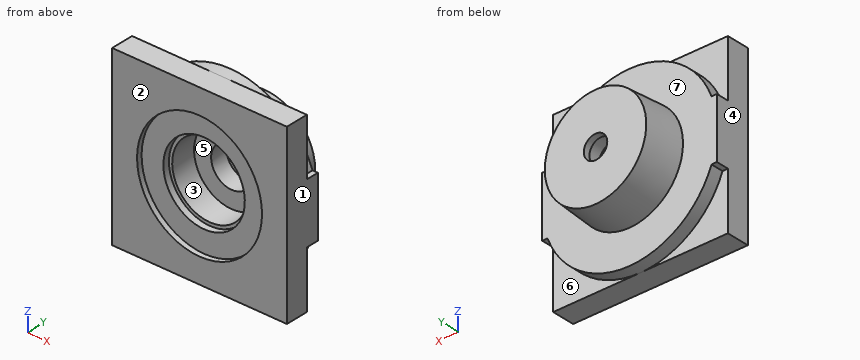
```python
from build123d import *

# Parameters (mm, degrees)
SKETCH1_W               = 7.01
SKETCH1_H               = 7.01
BOSS_EXTRUDE1_DEPTH     = 0.92
SKETCH2_R               = 3.505
BOSS_EXTRUDE2_DEPTH     = 0.83
SKETCH3_R               = 2.135
BOSS_EXTRUDE3_DEPTH     = 1.752116255
SKETCH4_R               = 2.085
CUT_EXTRUDE1_DEPTH      = 1
CUT_EXTRUDE2_DEPTH      = 7.069173606
CUT_EXTRUDE2_DEPTH_BACK = 7.069173606
SKETCH5_W               = 2.65
SKETCH5_H               = 2.65
SKETCH6_W               = 8.843273239
SKETCH6_H               = 10.721573241
SKETCH6_W_2             = 7.01
SKETCH6_H_2             = 7.01
SKETCH6_W_3             = 6
SKETCH6_H_3             = 6
CUT_EXTRUDE3_DEPTH      = 10
SKETCH7_W               = 8.855260717
SKETCH7_H               = 9.729262333
SKETCH7_R               = 3
CUT_EXTRUDE4_DEPTH      = 0.83
SKETCH8_W               = 2.771053774
SKETCH8_H               = 2.773686404
BOSS_EXTRUDE4_DEPTH     = 2.502116255
SKETCH9_R               = 0.554
CUT_EXTRUDE5_DEPTH      = 0.3
SKETCH10_R              = 0.47
CUT_EXTRUDE6_DEPTH      = 100
SKETCH11_R              = 1.501
CUT_EXTRUDE7_DEPTH      = 0.48
SKETCH12_R              = 0.817
CUT_EXTRUDE8_DEPTH      = 0.7
SKETCH14_R              = 0.582
CUT_EXTRUDE9_DEPTH      = 0.56
BOSS_EXTRUDE5_START     = 0.05
SKETCH15_R              = 0.554
SKETCH15_R_2            = 0.47
BOSS_EXTRUDE5_DEPTH     = 0.05
BOSS_EXTRUDE6_START     = 0.79
SKETCH16_R              = 2.085
SKETCH16_R_2            = 1.63
BOSS_EXTRUDE6_DEPTH     = 0.79
BOSS_EXTRUDE7_START     = 0.53
SKETCH17_R              = 1.63
SKETCH17_R_2            = 1.501
BOSS_EXTRUDE7_DEPTH     = 0.53
SKETCH18_R              = 2.572537364
SKETCH18_R_2            = 1.5
CUT_EXTRUDE10_DEPTH     = 1.752116255
BOSS_EXTRUDE8_START     = 0.21
SKETCH19_R              = 2.085
SKETCH19_R_2            = 1.705
BOSS_EXTRUDE8_DEPTH     = 0.21
SKETCH20_W              = 6.707027697
SKETCH20_H              = 11.442069063
SKETCH20_R              = 1.8
CUT_EXTRUDE11_DEPTH     = 0.83
SKETCH21_W              = 6.520255289
SKETCH21_H              = 15.458610975
SKETCH21_W_2            = 3.8
SKETCH21_H_2            = 3.8
CUT_EXTRUDE12_DEPTH     = 10
SKETCH23_W              = 6.99
SKETCH23_H              = 6.99
SKETCH23_W_2            = 3.502421246
SKETCH23_H_2            = 3.548313749
BOSS_EXTRUDE9_DEPTH     = 0.92
SKETCH24_W              = 6.057488838
SKETCH24_H              = 5.341048382
CUT_EXTRUDE14_DEPTH     = 0.13
SKETCH25_R              = 3.495
SKETCH25_R_2            = 1.679124266
BOSS_EXTRUDE10_DEPTH    = 0.83
SKETCH26_W              = 0.8
SKETCH26_H              = 2.36
BOSS_EXTRUDE11_DEPTH    = 0.83
SKETCH27_W              = 0.802423375
SKETCH27_H              = 2.36
BOSS_EXTRUDE12_DEPTH    = 0.83
SKETCH28_R              = 2.14
SKETCH28_R_2            = 1.325961915
BOSS_EXTRUDE13_DEPTH    = 1.622116255
SKETCH29_R              = 2.5
CUT_EXTRUDE15_DEPTH     = 0.21
SKETCH30_W              = 0.025
SKETCH30_H              = 0.83
BOSS_EXTRUDE14_DEPTH    = 0.4
SKETCH31_W              = 0.025
SKETCH31_H              = 0.83
BOSS_EXTRUDE15_DEPTH    = 0.4
SKETCH32_R              = 5.119404283
SKETCH32_R_2            = 2.14
CUT_EXTRUDE16_DEPTH     = 0.32
SKETCH33_W              = 6.584709795
SKETCH33_H              = 4.796866642
CUT_EXTRUDE17_DEPTH     = 0.37
SKETCH35_W              = 5.183427323
SKETCH35_H              = 5.029681598
SKETCH35_R              = 2.14
CUT_EXTRUDE18_DEPTH     = 1.572116
CUT_EXTRUDE18_DRAFT     = -4


with BuildPart() as part:
    # Sketch1 → Boss-Extrude1 (new body)
    with BuildSketch(Plane(origin=(0, 0, 0), x_dir=(1, 0, 0), z_dir=(0, 1, 0))):
        Rectangle(SKETCH1_W, SKETCH1_H)
    extrude(amount=BOSS_EXTRUDE1_DEPTH)

    # Sketch2 → Boss-Extrude2 (add)
    with BuildSketch(Plane(origin=(0, 0.92, 0), x_dir=(1, 0, 0), z_dir=(0, 1, 0))):
        with Locations(Location((0, 0, 0), (0, 0, 270))):
            Circle(SKETCH2_R)
    extrude(amount=BOSS_EXTRUDE2_DEPTH)

    # Sketch3 → Boss-Extrude3 (add)
    with BuildSketch(Plane(origin=(0, 1.75, 0), x_dir=(1, 0, 0), z_dir=(0, 1, 0))):
        with Locations(Location((0, 0, 0), (0, 0, 270))):
            Circle(SKETCH3_R)
    extrude(amount=BOSS_EXTRUDE3_DEPTH)

    # Sketch4 → Cut-Extrude1 (cut)
    with BuildSketch(Plane.XZ):
        with Locations(Location((0, 0, 0), (0, 0, 270))):
            Circle(SKETCH4_R)
    extrude(amount=-CUT_EXTRUDE1_DEPTH, mode=Mode.SUBTRACT)

    # Sketch5 → Cut-Extrude2 (cut, two sides: drawn at the far end of the back side and taken through both)
    with BuildSketch(Plane(origin=(0, 3.502116255, 0), x_dir=(1, 0, 0), z_dir=(0, 1, 0)).offset(-CUT_EXTRUDE2_DEPTH_BACK)):
        Rectangle(SKETCH5_W, SKETCH5_H)
    extrude(amount=CUT_EXTRUDE2_DEPTH + CUT_EXTRUDE2_DEPTH_BACK, mode=Mode.SUBTRACT)

    # Sketch6 → Cut-Extrude3 (cut)
    # profile 1 of 2: a face of its own
    with BuildSketch(Plane.XZ):
        with Locations((-0.050657098, -0.002715124)):
            Rectangle(SKETCH6_W, SKETCH6_H)
        Rectangle(SKETCH6_W_2, SKETCH6_H_2, mode=Mode.SUBTRACT)
    # profile 2 of 2: a face of its own
    with BuildSketch(Plane.XZ):
        Rectangle(SKETCH6_W_2, SKETCH6_H_2)
        Rectangle(SKETCH6_W_3, SKETCH6_H_3, mode=Mode.SUBTRACT)
    extrude(amount=-CUT_EXTRUDE3_DEPTH, mode=Mode.SUBTRACT)

    # Sketch7 → Cut-Extrude4 (cut)
    with BuildSketch(Plane(origin=(0, 1.75, 0), x_dir=(1, 0, 0), z_dir=(0, 1, 0))):
        with Locations((-0.111516438, -0.542198567)):
            Rectangle(SKETCH7_W, SKETCH7_H)
        with Locations(Location((0, 0, 0), (0, 0, 270))):
            Circle(SKETCH7_R, mode=Mode.SUBTRACT)
    extrude(amount=-CUT_EXTRUDE4_DEPTH, mode=Mode.SUBTRACT)

    # Sketch8 → Boss-Extrude4 (add)
    with BuildSketch(Plane.XZ.offset(-1)):
        with Locations((0.002668444, 0.023551669)):
            Rectangle(SKETCH8_W, SKETCH8_H)
    extrude(amount=-BOSS_EXTRUDE4_DEPTH)

    # Sketch9 → Cut-Extrude5 (cut)
    with BuildSketch(Plane(origin=(0, 3.502116255, 0), x_dir=(1, 0, 0), z_dir=(0, 1, 0))):
        with Locations(Location((0, 0, 0), (0, 0, 270))):
            Circle(SKETCH9_R)
    extrude(amount=-CUT_EXTRUDE5_DEPTH, mode=Mode.SUBTRACT)

    # Sketch10 → Cut-Extrude6 (cut)
    with BuildSketch(Plane(origin=(0, 3.202116255, 0), x_dir=(1, 0, 0), z_dir=(0, 1, 0))):
        with Locations(Location((0, 0, 0), (0, 0, 270))):
            Circle(SKETCH10_R)
    extrude(amount=-CUT_EXTRUDE6_DEPTH, mode=Mode.SUBTRACT)

    # Sketch11 → Cut-Extrude7 (cut)
    with BuildSketch(Plane.XZ.offset(-1)):
        with Locations(Location((0, 0, 0), (0, 0, 270))):
            Circle(SKETCH11_R)
    extrude(amount=-CUT_EXTRUDE7_DEPTH, mode=Mode.SUBTRACT)

    # Sketch12 → Cut-Extrude8 (cut)
    with BuildSketch(Plane.XZ.offset(-1.48)):
        with Locations(Location((0, 0, 0), (0, 0, 270))):
            Circle(SKETCH12_R)
    extrude(amount=-CUT_EXTRUDE8_DEPTH, mode=Mode.SUBTRACT)

    # Sketch14 → Cut-Extrude9 (cut)
    with BuildSketch(Plane.XZ.offset(-2.18)):
        with Locations(Location((0, 0, 0), (0, 0, 270))):
            Circle(SKETCH14_R)
    extrude(amount=-CUT_EXTRUDE9_DEPTH, mode=Mode.SUBTRACT)

    # Sketch15 → Boss-Extrude5 (add)
    with BuildSketch(Plane(origin=(0, 3.202116255, 0), x_dir=(1, 0, 0), z_dir=(0, 1, 0)).offset(BOSS_EXTRUDE5_START)):
        with Locations(Location((0, 0, 0), (0, 0, 270))):
            Circle(SKETCH15_R)
        with Locations(Location((0, 0, 0), (0, 0, 270))):
            Circle(SKETCH15_R_2, mode=Mode.SUBTRACT)
    extrude(amount=-BOSS_EXTRUDE5_DEPTH)

    # Sketch16 → Boss-Extrude6 (add)
    with BuildSketch(Plane.XZ.offset(-1).offset(BOSS_EXTRUDE6_START)):
        with Locations(Location((0, 0, 0), (0, 0, 270))):
            Circle(SKETCH16_R)
        with Locations(Location((0, 0, 0), (0, 0, 90))):
            Circle(SKETCH16_R_2, mode=Mode.SUBTRACT)
    extrude(amount=-BOSS_EXTRUDE6_DEPTH)

    # Sketch17 → Boss-Extrude7 (add)
    with BuildSketch(Plane.XZ.offset(-1).offset(BOSS_EXTRUDE7_START)):
        with Locations(Location((0, 0, 0), (0, 0, 90))):
            Circle(SKETCH17_R)
        with Locations(Location((0, 0, 0), (0, 0, 270))):
            Circle(SKETCH17_R_2, mode=Mode.SUBTRACT)
    extrude(amount=-BOSS_EXTRUDE7_DEPTH)

    # Sketch18 → Cut-Extrude10 (cut)
    with BuildSketch(Plane(origin=(0, 3.502116255, 0), x_dir=(1, 0, 0), z_dir=(0, 1, 0))):
        Circle(SKETCH18_R)
        with Locations(Location((0, 0, 0), (0, 0, 270))):
            Circle(SKETCH18_R_2, mode=Mode.SUBTRACT)
    extrude(amount=-CUT_EXTRUDE10_DEPTH, mode=Mode.SUBTRACT)

    # Sketch19 → Boss-Extrude8 (add)
    with BuildSketch(Plane.XZ.offset(-0.21).offset(BOSS_EXTRUDE8_START)):
        Circle(SKETCH19_R)
        with Locations(Location((0, 0, 0), (0, 0, 90))):
            Circle(SKETCH19_R_2, mode=Mode.SUBTRACT)
    extrude(amount=-BOSS_EXTRUDE8_DEPTH)

    # Sketch20 → Cut-Extrude11 (cut)
    with BuildSketch(Plane(origin=(0, 1.75, 0), x_dir=(1, 0, 0), z_dir=(0, 1, 0))):
        with Locations((0.104915626, 1.709559423)):
            Rectangle(SKETCH20_W, SKETCH20_H)
        with Locations(Location((0, 0, 0), (0, 0, 270))):
            Circle(SKETCH20_R, mode=Mode.SUBTRACT)
    extrude(amount=-CUT_EXTRUDE11_DEPTH, mode=Mode.SUBTRACT)

    # Sketch21 → Cut-Extrude12 (cut)
    with BuildSketch(Plane(origin=(0, 0.92, 0), x_dir=(1, 0, 0), z_dir=(0, 1, 0))):
        with Locations((-0.167365124, 0.45607417)):
            Rectangle(SKETCH21_W, SKETCH21_H)
        Rectangle(SKETCH21_W_2, SKETCH21_H_2, mode=Mode.SUBTRACT)
    extrude(amount=-CUT_EXTRUDE12_DEPTH, mode=Mode.SUBTRACT)

    # Sketch23 → Boss-Extrude9 (add)
    with BuildSketch(Plane.XZ):
        Rectangle(SKETCH23_W, SKETCH23_H)
        with Locations((-0.032460289, -0.038632405)):
            Rectangle(SKETCH23_W_2, SKETCH23_H_2, mode=Mode.SUBTRACT)
    extrude(amount=-BOSS_EXTRUDE9_DEPTH)

    # Sketch24 → Cut-Extrude14 (cut)
    with BuildSketch(Plane(origin=(0, 3.502116255, 0), x_dir=(1, 0, 0), z_dir=(0, 1, 0))):
        with Locations((0.48256212, -0.051480008)):
            Rectangle(SKETCH24_W, SKETCH24_H)
    extrude(amount=-CUT_EXTRUDE14_DEPTH, mode=Mode.SUBTRACT)

    # Sketch25 → Boss-Extrude10 (add)
    with BuildSketch(Plane(origin=(0, 0.92, 0), x_dir=(1, 0, 0), z_dir=(0, 1, 0))):
        with Locations(Location((0, 0, 0), (0, 0, 270))):
            Circle(SKETCH25_R)
        Circle(SKETCH25_R_2, mode=Mode.SUBTRACT)
    extrude(amount=BOSS_EXTRUDE10_DEPTH)

    # Sketch26 → Boss-Extrude11 (add)
    with BuildSketch(Plane(origin=(0, 1.75, 0), x_dir=(1, 0, 0), z_dir=(0, 1, 0))):
        with Locations((3.095, 0)):
            Rectangle(SKETCH26_W, SKETCH26_H)
    extrude(amount=-BOSS_EXTRUDE11_DEPTH)

    # Sketch27 → Boss-Extrude12 (add)
    with BuildSketch(Plane(origin=(0, 1.75, 0), x_dir=(1, 0, 0), z_dir=(0, 1, 0))):
        with Locations((-3.093788313, 0)):
            Rectangle(SKETCH27_W, SKETCH27_H)
    extrude(amount=-BOSS_EXTRUDE12_DEPTH)

    # Sketch28 → Boss-Extrude13 (add)
    with BuildSketch(Plane(origin=(0, 3.372116255, 0), x_dir=(1, 0, 0), z_dir=(0, 1, 0))):
        with Locations(Location((0, 0, 0), (0, 0, 270))):
            Circle(SKETCH28_R)
        Circle(SKETCH28_R_2, mode=Mode.SUBTRACT)
    extrude(amount=-BOSS_EXTRUDE13_DEPTH)

    # Sketch29 → Cut-Extrude15 (cut)
    with BuildSketch(Plane.XZ):
        with Locations(Location((0, 0, 0), (0, 0, 270))):
            Circle(SKETCH29_R)
    extrude(amount=-CUT_EXTRUDE15_DEPTH, mode=Mode.SUBTRACT)

    # Sketch30 → Boss-Extrude14 (add)
    with BuildSketch(Plane.ZY.offset(3.495)):
        with Locations((-1.1925, 1.335)):
            Rectangle(SKETCH30_W, SKETCH30_H)
        with Locations((1.1925, 1.335)):
            Rectangle(SKETCH30_W, SKETCH30_H)
    extrude(amount=-BOSS_EXTRUDE14_DEPTH)

    # Sketch31 → Boss-Extrude15 (add)
    with BuildSketch(Plane(origin=(3.495, 0, 0), x_dir=(0, 0, -1), z_dir=(1, 0, 0))):
        with Locations((-1.1925, 1.335)):
            Rectangle(SKETCH31_W, SKETCH31_H)
        with Locations((1.1925, 1.335)):
            Rectangle(SKETCH31_W, SKETCH31_H)
    extrude(amount=-BOSS_EXTRUDE15_DEPTH)

    # Sketch32 → Cut-Extrude16 (cut)
    with BuildSketch(Plane(origin=(0, 1.75, 0), x_dir=(1, 0, 0), z_dir=(0, 1, 0))):
        Circle(SKETCH32_R)
        with Locations(Location((0, 0, 0), (0, 0, 270))):
            Circle(SKETCH32_R_2, mode=Mode.SUBTRACT)
    extrude(amount=-CUT_EXTRUDE16_DEPTH, mode=Mode.SUBTRACT)

    # Sketch33 → Cut-Extrude17 (cut)
    with BuildSketch(Plane(origin=(0, 3.372116255, 0), x_dir=(1, 0, 0), z_dir=(0, 1, 0))):
        with Locations((0.213047648, -0.01757094)):
            Rectangle(SKETCH33_W, SKETCH33_H)
    extrude(amount=-CUT_EXTRUDE17_DEPTH, mode=Mode.SUBTRACT)


with BuildPart() as cut_extrude18_tool:
    # Sketch35 → Cut-Extrude18 (with draft: the straight prism first)
    with BuildSketch(Plane(origin=(0, 1.43, 0), x_dir=(1, 0, 0), z_dir=(0, 1, 0))):
        with Locations((0.01757094, -0.081265598)):
            Rectangle(SKETCH35_W, SKETCH35_H)
        Circle(SKETCH35_R, mode=Mode.SUBTRACT)
    extrude(amount=CUT_EXTRUDE18_DEPTH)
    # Cut-Extrude18: the draft: its side faces are tilted about the plane it starts from
    cut_extrude18_sides = [cut_extrude18_tool.faces().sort_by_distance(p)[0] for p in [
        (-2.574142721, 2.216058, 0.081265598),
        (0.01757094, 2.216058, 2.596106397),
        (2.609284602, 2.216058, 0.081265598),
        (0.01757094, 2.216058, -2.433575201),
        (-2.14, 2.216058, 0),
    ]]
    draft(cut_extrude18_sides, Plane(origin=(0, 1.43, 0), x_dir=(1, 0, 0), z_dir=(0, 1, 0)), CUT_EXTRUDE18_DRAFT)


with BuildPart() as part_1:
    add(part.part)

    # Cut-Extrude18: cut by cut_extrude18_tool
    add(cut_extrude18_tool.part, mode=Mode.SUBTRACT)


solid = part_1.part
```
Work out the finished part from the listing and answer in its coordinate system (mm). Face numbers are marked on the shaded views. A direction names the side the tool comes from. Give positions to 0.01 mm unless a question says otherwise; leave off trailing zeros. Write each loop counter-clockwise with the first axis right and the second up, starting at its lowest first coordinate (ties: lowest second). Pieces come first, ordered by that corner, then holes. Notation, with made-up numbers: (47.25, 60) -> (73.25, 60) arc R16 ccw to (73.25, 81) -> close; hole circle Ø4 at (38.25, 71.25). An arc over 180 degrees is marked (long way). Write item = value, one per line.
Q1. Section D-D on y = 0.3 is taken. Determine the outline of the cut face in (x, z) (3 decimals).
Computed values:
outline = (-3.495, -3.495) -> (3.495, -3.495) -> (3.495, 3.495) -> (-3.495, 3.495) -> close; hole circle Ø3.26 at (0, 0)
Q2. For a pull along X with two mould halves and no side action, classify the marked faces 1, 2, 3 and 4 as pulls with the +X half, pulls with the -X half, needs draft (parallel to the pull), parting line crosses it, or undercut.
Computed values:
face_1 = pulls with the +X half
face_2 = needs draft
face_3 = undercut
face_4 = pulls with the -X half
Q3. Section B-B on y = 1.3 is taken. Determine the outline of the cut face in (x, z) (3 decimals), and give its area (3 significant figures).
Computed values:
outline = (-3.495, -1.205) -> (-3.281, -1.205) arc R3.495 ccw to (3.281, -1.205) -> (3.495, -1.205) -> (3.495, 1.205) -> (3.281, 1.205) arc R3.495 ccw to (-3.281, 1.205) -> (-3.495, 1.205) -> close; hole circle Ø3.002 at (0, 0)
area = 31.6 mm^2
Q4. A tool of negligible diameter and unlimited length cuts with its end or side. For the marked faces 5, 6 and 7, from which of +Z, -Z, +X, -X, +Y, -Y can it reach the whole face along a straight path? Write none if from no direction.
Computed values:
face_5 = -Y
face_6 = -Z, +X, +Y
face_7 = +Y
Q5. Section C-C on x = -3 is taken. Determine the outline of the cut face in (y, z) (3 decimals), and give its area (3 significant figures).
Computed values:
outline = (0, -3.495) -> (0.92, -3.495) -> (0.92, -1.793) -> (1.43, -1.793) -> (1.43, 1.793) -> (0.92, 1.793) -> (0.92, 3.495) -> (0, 3.495) -> close
area = 8.26 mm^2
Q6. Consider line 1 along X through (y, z) = (0.35, 0) (3 decimals); line 2 along Y through (x, z) = (-1.75, 1.75); line 3 along Y through (x, z) = (-0.25, 1). Determine where each line is inside the solid, lowest interval first.
Computed values:
line_1 = -3.495 to -1.63, 1.63 to 3.495
line_2 = 0.21 to 1.43
line_3 = 1.48 to 3
Q7. Flat-ended cylindrical pins translate along their axes: pin 1 Ø1.8 at (x, z) = (0.5, 0) entering from -Y; pin 2 Ø1.5 at (x, y) = (1, 2.5) entering from +Z; pin 3 Ø1.1 at (x, z) = (2, -2.5) entering from +Y. Find the tip coordinate at first contact, or state that the pin passes through.
Computed values:
pin_1 = 1.48
pin_2 = 2.06
pin_3 = 1.43
